Geometry check sheet. Reference: the model listing, model coordinates, mm. Face numbers are marked on the shaded views. Round coordinates to 2 decimals unless told otherwise and drop trailing zeros. Loops run counter-clockwise (first coordinate to the right, second up) from the corner with the lowest first, then second, coordinate; pieces in that order, holes last. Notation, with made-up numbers: (76, 28) - (111, 28) arc R23 ccw to (111, 43) - close; hole circle Ø2 at (4, -14.75). An arc over 180 degrees is marked (long way). Write item = value, one per line.
```python
from build123d import *

# Parameters (mm, degrees)
F0_W     = 609.6
F0_H     = 381
F1_DEPTH = 19.05
F2_SIZE2 = 27.2352378905
F2_SIZE  = 12.7
F3_W     = 50.8
F3_H     = 889
F4_DEPTH = 25.4
F5_W     = 6.35
F5_H     = 50.8
F6_DEPTH = 25.4
F7_T     = -0.0254


with BuildPart() as f1:
    # F0 (on Top) → F1 (new body)
    with BuildSketch(Plane.XY):
        Rectangle(F0_W, F0_H)
    extrude(amount=F1_DEPTH)

    # F2
    f2_edges = [f1.edges().sort_by_distance(p)[0] for p in [
        (0, -190.5, 0),
        (304.8, 0, 0),
        (0, 190.5, 0),
        (-304.8, 0, 0),
    ]]
    chamfer(f2_edges, length=F2_SIZE, length2=F2_SIZE2)

    # F3 (on Right) → F4 (join, symmetric)
    with BuildSketch(Plane.YZ):
        Rectangle(F3_W, F3_H)
    extrude(amount=F4_DEPTH, both=True)

    # F5 (on face) → F6 (intersect)
    with BuildSketch(Plane.YZ.offset(25.4)):
        with Locations((9.525, 406.4)):
            Rectangle(F5_W, F5_H)
    extrude(amount=-F6_DEPTH, mode=Mode.INTERSECT)

    # F7
    f7_openings = [f1.faces().sort_by_distance(p)[0] for p in [
        (25.4, 9.525, 406.4),
    ]]
    offset(amount=F7_T, openings=f7_openings)


solid = f1.part
```
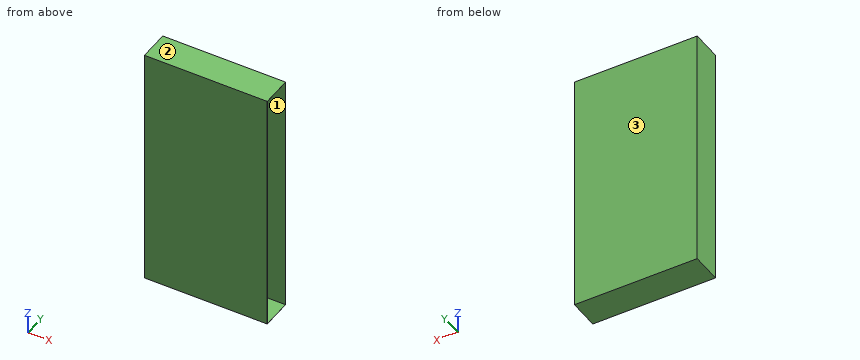
(1) Section check A-A (x = 18.5). Enter the section's corners in (y, z).
Answers follow:
outline = (6.35, 381) - (12.7, 381) - (12.7, 431.8) - (6.35, 431.8) - close; hole (6.38, 381.03) - (12.67, 381.03) - (12.67, 431.77) - (6.38, 431.77) - close
(2) Gauge pin test, flat end, axial feed: pin 1 (2 mm diameter, centred on y = 7.5, z = 400.5, fed in from +X). Record the tip position at first contact, or that the pin passes through.
Answers follow:
pin_1 = 0.03
(3) Mould release check, pull along Y, two halves, no side actions. Record for the marked faces 1, 2 and 3: pulls with the +Y half, pulls with the -Y half, needs draft (parallel to the pull), parting line crosses it, or undercut.
Answers follow:
face_1 = undercut
face_2 = needs draft
face_3 = pulls with the +Y half
